Input: part model. Units: mm. Frame: model coordinates. A direction names the side the tool comes from. Give positions to 0.01 mm unless a question says otherwise; leave off trailing zeros. Loops run counter-clockwise (first coordinate to the right, second up) from the corner with the lowest first, then second, coordinate; pieces in that order, holes last. Notation, with made-up numbers: (-4.75, 32.5) - (26.25, 32.5) arc R21 cw to (26.25, 38.5) - close; hole circle Ø1 at (-34, -1.75). An arc over 180 degrees is marked (long way). One line per item, written item: value.
from build123d import *

# Parameters (mm, degrees)
EXTRUDE_2_DEPTH     = 1.7
CUT_EXTRUDE_START   = 0.3
SKETCH_3_W          = 1.35
SKETCH_3_H          = 1.35
CUT_EXTRUDE_2_DEPTH = 1
SCALE_1_SCALE       = 10


with BuildPart() as part:
    # 스케치1 → 보스-돌출2 (new body)
    with BuildSketch(Plane.XY):
        Polygon((-3.15, 0), (3.15, 0), (1.709287021, 0.5), (1.279556076, 1), (-1.279556076, 1), (-1.709287021, 0.5), align=None)
    extrude(amount=EXTRUDE_2_DEPTH)

    # 스케치3 → 컷-돌출2 (cut)
    with BuildSketch(Plane(origin=(0, 1, 0), x_dir=(1, 0, 0), z_dir=(0, 1, 0)).offset(CUT_EXTRUDE_START)):
        with Locations((-0.002241196, -0.851457908)):
            Rectangle(SKETCH_3_W, SKETCH_3_H)
    extrude(amount=-CUT_EXTRUDE_2_DEPTH, mode=Mode.SUBTRACT)


with BuildPart() as part_1:
    # 축척1: scaled about (0.000529957, 0.366302106, 0.84965526)
    add(part.part.scale(SCALE_1_SCALE).moved(Location((-0.004769613, -3.296718954, -7.64689734))))


solid = part_1.part
Item 1: Pin query (flat end, axial travel): P1, Ø3.5, axis at y = 4, z = 2, coming from the -X side. Return the tip coordinate at first contact, or that it passes through.
Verdict:
P1: stops at x = -16.63
Item 2: Draft query along X for faces 3 (the face through (0, 6.703, 8)), 4 (the face through (24.39, -0.83, 0.73)), 5 (the face through (-6.777, 3, 1)). Return one class per face: pulls with the +X half, pulls with the -X half, needs draft (parallel to the pull), parting line crosses it, or undercut.
Verdict:
face 3: needs draft
face 4: pulls with the +X half
face 5: undercut
Item 3: Material intervals for L1, parallel to Z at x = -6, y = 1.25; L2, parallel to X at y = 4.75, z = 5.25; L3, parallel to X at y = 6, z = 2, sorted ascending.
Verdict:
L1: z = -7.65 to -5.88, 7.62 to 9.35
L2: x = -14.48 to -6.78, 6.72 to 14.47
L3: x = -13.4 to -6.78, 6.72 to 13.4
Item 4: Section A-A, the plane y = 3. Output: boundary loops of the cut face in (x, z), and give its area (3 significant figures).
Verdict:
outline: (-15.98, -7.65) - (15.97, -7.65) - (15.97, 9.35) - (-15.98, 9.35) - close; hole (-6.78, -5.88) - (6.72, -5.88) - (6.72, 7.62) - (-6.78, 7.62) - close
area: 361 mm^2
Item 5: Access query for faces 1 (the face through (-24.2, -0.76, 0.73)), 2 (the face through (0, 3, -5.882)). Directions: +Z, -Z, +X, -X, +Y, -Y. A direction counts if a zero-diameter tool reaches every point of the face in a straight line with its end or side. Return the directions, or none.
Verdict:
face 1: +Z, -Z, -X, +Y
face 2: +Y
Item 6: Section C-C, the plane x = -6. Output: boundary loops of the cut face in (y, z).
Verdict:
outline: (-3.3, -7.65) - (6.7, -7.65) - (6.7, -5.88) - (-0.3, -5.88) - (-0.3, 7.62) - (6.7, 7.62) - (6.7, 9.35) - (-3.3, 9.35) - close
Item 7: Section D-D, the plane y = 0.25. Output: boundary loops of the cut face in (x, z).
Verdict:
outline: (-21.29, -7.65) - (21.28, -7.65) - (21.28, 9.35) - (-21.29, 9.35) - close; hole (-6.78, -5.88) - (6.72, -5.88) - (6.72, 7.62) - (-6.78, 7.62) - close
Item 8: Section B-B, the plane z = -2.75. Output: boundary loops of the cut face in (x, y), and give its area (3 significant figures).
Verdict:
outline: (-31.5, -3.3) - (31.5, -3.3) - (17.09, 1.7) - (12.79, 6.7) - (6.72, 6.7) - (6.72, -0.3) - (-6.78, -0.3) - (-6.78, 6.7) - (-12.8, 6.7) - (-17.1, 1.7) - close
area: 298 mm^2
